Study the drawing (mm; zero at the part's minimum x, y, z) and answer. A direction names the side the tool comes from. Coordinates: 2 decimals unless noted, no trailing zeros. Write each loop counter-clockwise with the first axis right and the second up, starting at its lowest first coordinate (ties: lowest second). Pieces come first, ordered by that corner, then holes. Notation, with made-up numbers: M 56,85 L 64,85 A23 ccw 64,112 Z; hole C 57.25,63 d7. An arc over 180 degrees is marked long. Answer as a JSON object with one key per item and string values. Group by question number.
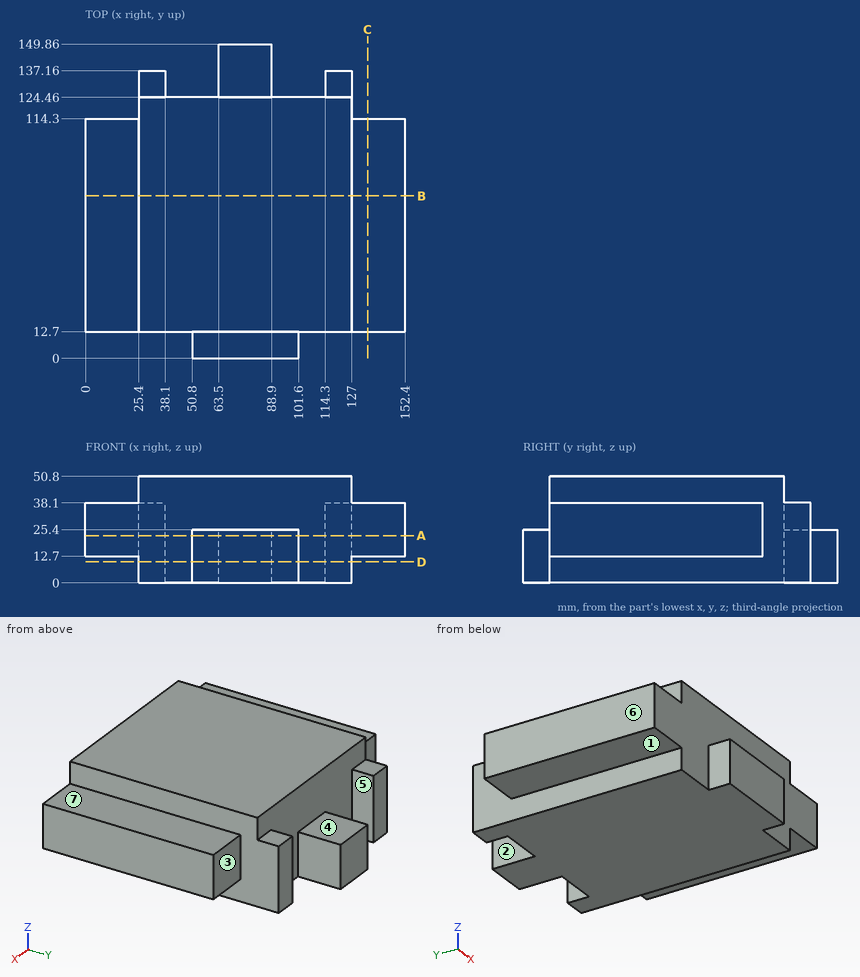
Item 1: A tool of negligible diameter and unlimited length cuts with its end or side. For the marked faces 1, 2, 3 and 4, from which of +Z, -Z, +X, -X, +Y, -Y can it reach the whole face along a straight path? Write none if from no direction.
Item 2: For a pull along X with two mould halves and no side action, classify the marked faces 5, 6 and 7 as +X half, -X half, draft (parallel to the pull), parting line (faces both ways), or undercut.
Item 3: A cutting plane is placed at B-B, the plane y = 77.5. Write down the section's boundary in (x, z), and give its area (3 significant figures).
Item 4: A cutting plane is placed at D-D, the plane z = 10. Write down the section's boundary in (x, y).
Item 5: Consider L1, parallel to Z at x = 129.5, y = 15; L2, parallel to X at y = 49, z = 8; L3, parallel to Y at x = 35, z = 3. Determine where each line is inside the solid, lowest interval first. Write a range as from..to.
Item 6: A cutting plane is placed at A-A, the plane z = 22.5. Write down the section's boundary in (x, y), and give its area (3 significant figures).
Item 7: Flat-ended cylindrical pins translate along their axes: pin 1 Ø7.5 at (y, z) = (137, 12) entering from +X; pin 2 Ø14 at (y, z) = (129, 17.5) entering from -X; pin 3 Ø6 at (x, z) = (26, 32) entering from -Y. Find the tip coordinate at first contact, or state that the pin passes through.
Item 8: A cutting plane is placed at C-C, the plane x = 134.5. Write down the section's boundary in (y, z).
Answer:
{
 "1": {"face 1": "-Z, -X, +Y, -Y", "face 2": "+Z, -Z, +Y", "face 3": "+Z, -Z, +X, +Y", "face 4": "+Z, +Y"},
 "2": {"face 5": "undercut", "face 6": "-X half", "face 7": "draft"},
 "3": {"outline": "M 0,12.7 L 25.4,12.7 L 25.4,0 L 127,0 L 127,12.7 L 152.4,12.7 L 152.4,38.1 L 127,38.1 L 127,50.8 L 25.4,50.8 L 25.4,38.1 L 0,38.1 Z", "area": "6,450 mm2"},
 "4": {"outline": "M 25.4,12.7 L 50.8,12.7 L 50.8,0 L 101.6,0 L 101.6,12.7 L 127,12.7 L 127,137.16 L 114.3,137.16 L 114.3,124.46 L 88.9,124.46 L 88.9,149.86 L 63.5,149.86 L 63.5,124.46 L 38.1,124.46 L 38.1,137.16 L 25.4,137.16 Z"},
 "5": {"L1": "12.7..38.1", "L2": "25.4..127", "L3": "12.7..137.16"},
 "6": {"outline": "M 0,12.7 L 50.8,12.7 L 50.8,0 L 101.6,0 L 101.6,12.7 L 152.4,12.7 L 152.4,114.3 L 127,114.3 L 127,137.16 L 114.3,137.16 L 114.3,124.46 L 88.9,124.46 L 88.9,149.86 L 63.5,149.86 L 63.5,124.46 L 38.1,124.46 L 38.1,137.16 L 25.4,137.16 L 25.4,114.3 L 0,114.3 Z", "area": "18,100 mm2"},
 "7": {"pin 1": "x = 127", "pin 2": "x = 25.4", "pin 3": "y = 12.7"},
 "8": {"outline": "M 12.7,12.7 L 114.3,12.7 L 114.3,38.1 L 12.7,38.1 Z"}
}
